Part model, mm, in its own coordinate system. Give positions to 0.01 mm unless a question says otherwise; leave off trailing zeros. Write each loop counter-clockwise with the first axis right and the second up, starting at its lowest first coordinate (ties: lowest second). Pieces come first, ordered by that corner, then holes.
```python
from build123d import *

# Parameters (mm, degrees)
F1_DEPTH = 25.4
F2_DEPTH = 25.4
F3_DEPTH = 25.4
F4_DEPTH = 25.4
F6_DEPTH = 50.8
F8_DEPTH = 50.8


with BuildPart() as f1:
    # F0 (on Front) → F1 (new body)
    with BuildSketch(Plane.XZ):
        Polygon((-25.4, 25.4), (-25.4, -25.4), (0, 0), align=None)
    extrude(amount=F1_DEPTH)

    # F0 (on Front) → F2 (join)
    with BuildSketch(Plane.XZ):
        Polygon((0, 0), (25.4, 25.4), (-25.4, 25.4), align=None)
    extrude(amount=F2_DEPTH)

    # F0 (on Front) → F3 (join)
    with BuildSketch(Plane.XZ):
        Polygon((0, 0), (25.4, -25.4), (25.4, 25.4), align=None)
    extrude(amount=F3_DEPTH)

    # F0 (on Front) → F4 (join)
    with BuildSketch(Plane.XZ):
        Polygon((-25.4, -25.4), (25.4, -25.4), (0, 0), align=None)
    extrude(amount=F4_DEPTH)

    # F5 (on face) → F6 (cut)
    with BuildSketch(Plane(origin=(0, 0, -25.4), x_dir=(1, 0, 0), z_dir=(0, 0, -1))):
        Polygon((-25.4, 0), (0, 25.4), (-25.4, 25.4), align=None)
    extrude(amount=-F6_DEPTH, mode=Mode.SUBTRACT)

    # F7 (on face) → F8 (cut)
    with BuildSketch(Plane.XY.offset(25.4)):
        Polygon((25.4, 0), (0, -25.4), (25.4, -25.4), align=None)
    extrude(amount=-F8_DEPTH, mode=Mode.SUBTRACT)


solid = f1.part
```
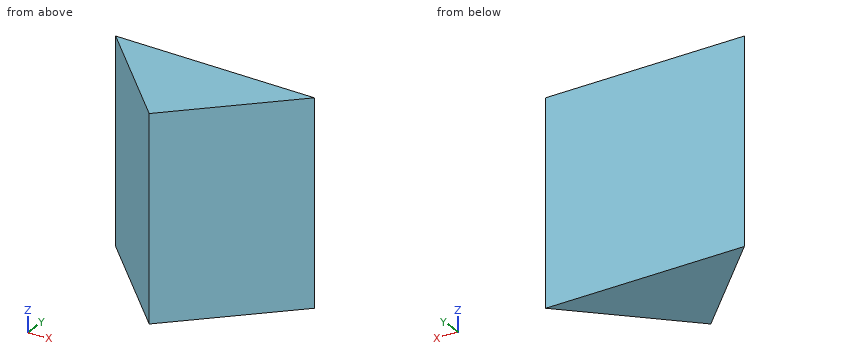
1) Saw through at B-B, the plane y = -3. Write the cut outline in (x, z), then the cut area to 3 significant figures.
Answers follow:
outline: (-22.4, -25.4) - (22.4, -25.4) - (22.4, 25.4) - (-22.4, 25.4) - close
area: 2,280 mm2
2) Saw through at A-A, the plane x = 10.5. Write the cut outline in (y, z).
Answers follow:
outline: (-14.9, -25.4) - (0, -25.4) - (0, 25.4) - (-14.9, 25.4) - close
3) Wall check: L1, parallel to X at y = -8.5, z = 14.5; L2, parallel to Y at x = -17.5, z = -15; L3, parallel to X at y = -21, z = -1. Give the ranges that are in metal, low to high.
Answers follow:
L1: x = -16.9 to 16.9
L2: y = -7.9 to 0
L3: x = -4.4 to 4.4
4) Pin check, flat tips, straight feed: pin 1 Ø5 at (y, z) = (-19.5, -5) entering from -X; pin 2 Ø8 at (y, z) = (-16, -13) entering from +X; pin 3 Ø1 at (y, z) = (-12, 9) entering from -X. Stop position of each tip, or through.
Answers follow:
pin 1: stops at x = -8.4
pin 2: stops at x = 13.4
pin 3: stops at x = -13.9
5) Saw through at C-C, the plane z = 16. Write the cut outline in (x, y).
Answers follow:
outline: (-25.4, 0) - (0, -25.4) - (25.4, 0) - close
